Source: CAD feature listing. Evaluate the final solid. Frame: model axes, mm. A direction names the side the tool comes from. Coordinates: 2 decimals unless noted, no trailing zeros. Loops run counter-clockwise (first coordinate to the right, second up) from the corner with the lowest first, then second, coordinate; pieces in that order, holes last.
Item 1: Line query: probe 1 along X at (y, z) = (9.25, 0); probe 2 along Z at (x, y) = (26, 3.25); probe 3 along Z at (x, y) = (7, 10.75). Output: solid intervals per line, ascending.
Item 2: Section query A-A, the plane x = 0. Return the cut outline in (y, z).
Item 3: Reachability of faces 5 (the cylindrical face through (1.3, 6.16, -29.62)), 6 (the cylindrical face through (-29.775, 7.43, -6.612)) from +Z, -Z, +X, -X, +Y, -Y: full face, straight path, thin tool, end or side. Return the list, or none.
Item 4: Pin query (flat end, axial travel): pin 1 Ø1.5 at (y, z) = (9.5, -20) entering from +X; pin 2 Ø6 at (x, y) = (22.5, 11) entering from -Z; pin 3 Ø3 at (y, z) = (2, -8.5) entering from +X. Return the tip coordinate at first contact, or that it passes through.
Item 5: Section query C-C, the plane y = 4.25. Return the cut outline in (x, z).
Item 6: Pull-direction query (X, two-part tool) for faces 1 (the flat face through (29, 2.5, 10)), 2 (the cylindrical face through (-14.17, 6.16, 34.18)), 3 (the cylindrical face through (10.633, 7.43, 33.765)), 4 (the flat face through (-33, 12.5, 14)); classes: +X half, -X half, draft (parallel to the pull), parting line (faces both ways), or undercut.
Item 7: Section query B-B, the plane z = 0. Return the cut outline in (x, y).
```python
from build123d import *

# Parameters (mm, degrees)
CROQUIS1_R              = 37
CROQUIS1_R_2            = 29.65
SALIENTE_EXTRUIR1_DEPTH = 2.5
CROQUIS2_R              = 37
CROQUIS2_R_2            = 35.4
CROQUIS2_R_3            = 30.5
CROQUIS2_R_4            = 29.65
SALIENTE_EXTRUIR2_DEPTH = 10


with BuildPart() as part:
    # Croquis1 → Saliente-Extruir1 (new body)
    with BuildSketch(Plane(origin=(0, 0, 0), x_dir=(1, 0, 0), z_dir=(0, 1, 0))):
        with Locations(Location((0, 0, 0), (0, 0, 270))):
            Circle(CROQUIS1_R)
        with Locations(Location((0, 0, 0), (0, 0, 270))):
            Circle(CROQUIS1_R_2, mode=Mode.SUBTRACT)
    extrude(amount=SALIENTE_EXTRUIR1_DEPTH)

    # Croquis2 → Saliente-Extruir2 (add)
    # profile 1 of 2: a face of its own
    with BuildSketch(Plane(origin=(0, 2.5, 0), x_dir=(1, 0, 0), z_dir=(0, 1, 0))):
        with Locations(Location((0, 0, 0), (0, 0, 270))):
            Circle(CROQUIS2_R)
        with Locations(Location((0, 0, 0), (0, 0, 270))):
            Circle(CROQUIS2_R_2, mode=Mode.SUBTRACT)
    # profile 2 of 2: a face of its own
    with BuildSketch(Plane(origin=(0, 2.5, 0), x_dir=(1, 0, 0), z_dir=(0, 1, 0))):
        with Locations(Location((0, 0, 0), (0, 0, 270))):
            Circle(CROQUIS2_R_3)
        with Locations(Location((0, 0, 0), (0, 0, 270))):
            Circle(CROQUIS2_R_4, mode=Mode.SUBTRACT)
    extrude(amount=SALIENTE_EXTRUIR2_DEPTH)


solid = part.part
```
Verdict:
1. probe 1: x = -37 to -35.4, -30.5 to -29.65, 29.65 to 30.5, 35.4 to 37
1. probe 2: z = -26.32 to -24.02, -15.95 to -14.25, 14.25 to 15.95, 24.02 to 26.32
1. probe 3: z = -36.33 to -34.7, -29.69 to -28.81, 28.81 to 29.69, 34.7 to 36.33
2. outline: (0, -37) - (12.5, -37) - (12.5, -35.4) - (2.5, -35.4) - (2.5, -30.5) - (12.5, -30.5) - (12.5, -29.65) - (0, -29.65) - close; (0, 29.65) - (12.5, 29.65) - (12.5, 30.5) - (2.5, 30.5) - (2.5, 35.4) - (12.5, 35.4) - (12.5, 37) - (0, 37) - close
3. face 5: +Y, -Y
3. face 6: +Y
4. pin 1: stops at x = 31.6
4. pin 2: stops at z = -31.44
4. pin 3: stops at x = 36.33
5. outline: circle Ø74 at (0, 0); circle Ø61 at (0, 0); hole circle Ø70.8 at (0, 0); hole circle Ø59.3 at (0, 0)
6. face 1: undercut
6. face 2: parting line
6. face 3: undercut
6. face 4: draft
7. outline: (-37, 0) - (-29.65, 0) - (-29.65, 12.5) - (-30.5, 12.5) - (-30.5, 2.5) - (-35.4, 2.5) - (-35.4, 12.5) - (-37, 12.5) - close; (29.65, 0) - (37, 0) - (37, 12.5) - (35.4, 12.5) - (35.4, 2.5) - (30.5, 2.5) - (30.5, 12.5) - (29.65, 12.5) - close
